from build123d import *

# Parameters (mm, degrees)
F0_W     = 38.1
F0_H     = 38.1
F1_DEPTH = 38.1
F6_DEPTH = 38.1


with BuildPart() as f1:
    # F0 (on Front) → F1 (new body)
    with BuildSketch(Plane.XZ):
        with Locations((19.05, 19.05)):
            Rectangle(F0_W, F0_H)
    extrude(amount=F1_DEPTH)

    # F5 (on face) → F6 (cut)
    with BuildSketch(Plane.YZ.offset(38.1)):
        Polygon((-31.75, 38.1), (-38.1, 38.1), (-38.1, 0), align=None)
        Polygon((-12.7, 38.1), (-25.4, 38.1), (-19.05, 22.225), align=None)
        Polygon((-6.35, 38.1), (0, 0), (0, 38.1), align=None)
        Polygon((-26.67, 17.5525732338), (-31.75, 0), (-6.35, 0), (-11.43, 17.5525732338), (-16.51, 9.525), (-21.59, 9.525), align=None)
    extrude(amount=-F6_DEPTH, mode=Mode.SUBTRACT)


solid = f1.part
Input: part model. Units: mm. Frame: model coordinates. A direction names the side the tool comes from. Give positions to 0.01 mm unless a question says otherwise; leave off trailing zeros. Write each loop counter-clockwise with the first axis right and the second up, starting at its lowest first coordinate (ties: lowest second). Pieces come first, ordered by that corner, then holes.
Q1. First-contact query: P1, Ø4, axis at x = 9, z = 9, coming from the -Y side; P2, Ø6, axis at x = 28.5, z = 23, coming from the -Y side; P3, Ø6, axis at x = 30.5, z = 4, coming from the +Y side. Flat tips, straight axial feed; report the tip coordinate or a pass-through.
Q2. Material intervals for probe 1 along Y at (x, z) = (22, 16); probe 2 along Y at (x, z) = (18, 28.5); probe 3 along Y at (x, z) = (25, 28), sorted ascending.
Q3. Section A-A, the plane z = 31.5. Output: boundary loops of the cut face in (x, y).
Q4. Pull-direction query (Y, two-part tool) for faces 4 (the face through (19.317, -8.854, 8.653)), 5 (the face through (19.32, -34.97, 18.78)), 6 (the face through (0, -19, 19)); classes: pulls with the +Y half, pulls with the -Y half, needs draft (parallel to the pull), parting line crosses it, or undercut.
Q5. Set-up query: faces 1 (the face through (38.1, -19, 19)), 2 (the face through (19, -19, 9.525)), 3 (the face through (19.32, -22.27, 30.27)). Return all of +Z, -Z, +X, -X, +Y, -Y with unobstructed straight access to the full face (end or side cutting, diameter ignored); none if empty.
Q6. Section B-B, the plane x = 24.5. Output: boundary loops of the cut face in (y, z) (3 decimals).
Q7. Section C-C, the plane z = 14.5. Output: boundary loops of the cut face in (x, y).
Q8. Section D-D, the plane y = -4. Output: boundary loops of the cut face in (x, z).
Filled in:
1. P1: stops at y = -36.93
1. P2: stops at y = -34.77
1. P3: stops at y = -0.17
2. probe 1: y = -35.43 to -27.12, -25.69 to -12.41, -10.98 to -2.67
2. probe 2: y = -33.35 to -21.56, -16.54 to -4.75
2. probe 3: y = -33.43 to -21.36, -16.74 to -4.67
3. outline: (0, -32.85) - (38.1, -32.85) - (38.1, -22.76) - (0, -22.76) - close; (0, -15.34) - (38.1, -15.34) - (38.1, -5.25) - (0, -5.25) - close
4. face 4: undercut
4. face 5: pulls with the -Y half
4. face 6: needs draft
5. face 1: +Z, -Z, +X, +Y, -Y
5. face 2: -Z, +X, -X
5. face 3: +Z, +X, -X
6. outline: (-38.1, 0) - (-31.75, 0) - (-26.67, 17.553) - (-21.59, 9.525) - (-16.51, 9.525) - (-11.43, 17.553) - (-6.35, 0) - (0, 0) - (-6.35, 38.1) - (-12.7, 38.1) - (-19.05, 22.225) - (-25.4, 38.1) - (-31.75, 38.1) - close
7. outline: (0, -35.68) - (38.1, -35.68) - (38.1, -27.55) - (0, -27.55) - close; (0, -24.74) - (38.1, -24.74) - (38.1, -13.36) - (0, -13.36) - close; (0, -10.55) - (38.1, -10.55) - (38.1, -2.42) - (0, -2.42) - close
8. outline: (0, 0) - (38.1, 0) - (38.1, 24) - (0, 24) - close
